Answer from the drawing. Dimensions are ordinates in mm from the lowest x, y and z of the part. Round coordinates to 2 decimals unless told otherwise and drop trailing zeros. Loops run counter-clockwise (first coordinate to the right, second up) from the corner with the lowest first, then second, coordinate; pieces in that order, holes last.
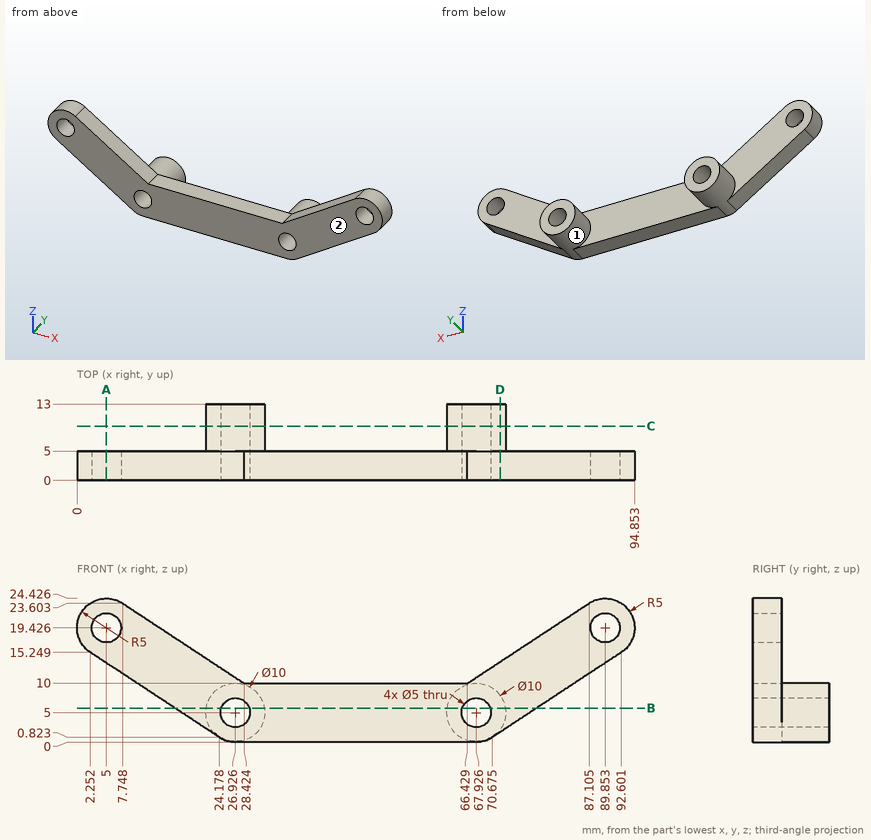
1. Find section D-D (x = 72). Write down the section's boundary in (y, z) (1 decimal).
Answer key:
outline: (0, 1.7) - (5, 1.7) - (5, 2.1) - (13, 2.1) - (13, 7.9) - (5, 7.9) - (5, 13.7) - (0, 13.7) - close
2. Find section B-B (z = 5.75). Write down the section's boundary in (x, y).
Answer key:
outline: (16.69, 0) - (24.54, 0) - (24.54, 13) - (21.98, 13) - (21.98, 5) - (16.69, 5) - close; (29.31, 0) - (65.54, 0) - (65.54, 13) - (62.98, 13) - (62.98, 5) - (31.87, 5) - (31.87, 13) - (29.31, 13) - close; (70.31, 0) - (78.16, 0) - (78.16, 5) - (72.87, 5) - (72.87, 13) - (70.31, 13) - close
3. Find section C-C (y = 9.25). Write down the section's boundary in (x, z), then the cut area to 3 significant figures.
Answer key:
outline: circle Ø10 at (26.93, 5); circle Ø10 at (67.93, 5); hole circle Ø5 at (26.93, 5); hole circle Ø5 at (67.93, 5)
area: 118 mm2
4. Given pin 1 (1 mm diameter, centred on x = 16.5, z = 13, fed in from +Y); pin 2 (1.5 mm diameter, centred on x = 42, y = 3, fed in from +Z); pin 3 (5 mm diameter, centred on x = 15, y = 1.5, fed in from +Z), each flat-ended and moving along its own axis, determine where each tip first touches the part or whether it passes through.
Answer key:
pin 1: stops at y = 5
pin 2: stops at z = 10
pin 3: stops at z = 20.48
5. Consider probe 1 along X at (y, z) = (6.25, 5); probe 2 along X at (y, z) = (4.5, 6) (1 decimal); probe 3 along X at (y, z) = (12.75, 3) (1 decimal). Determine where each line is inside the solid, lowest interval first.
Answer key:
probe 1: x = 21.93 to 24.43, 29.43 to 31.93, 62.93 to 65.43, 70.43 to 72.93
probe 2: x = 16.3 to 24.6, 29.2 to 65.6, 70.2 to 78.5
probe 3: x = 22.3 to 25.4, 28.4 to 31.5, 63.3 to 66.4, 69.4 to 72.5
6. Find section A-A (x = 5). Write down the section's boundary in (y, z).
Answer key:
outline: (0, 13.44) - (5, 13.44) - (5, 16.93) - (0, 16.93) - close; (0, 21.93) - (5, 21.93) - (5, 24.43) - (0, 24.43) - close
7. Determine the mould class of the marked faces 1 and 2 for opening direction X: +X half, -X half, draft (parallel to the pull), parting line (faces both ways), or undercut.
Answer key:
face 1: undercut
face 2: draft
